Input: part model. Units: mm. Frame: model coordinates. A direction names the side the tool comes from. Give positions to 0.01 mm unless a question says otherwise; leave off trailing zeros. Loops run counter-clockwise (first coordinate to the right, second up) from the corner with the lowest first, then second, coordinate; pieces in that order, holes last. Notation, with made-up numbers: (47, -35) -> (77, -35) arc R15 ccw to (77, -17) -> close; hole circle Ø7 at (-7.75, 46.5). An arc over 180 degrees is marked (long way). Answer as a JSON object with one key per item and string values.
```python
from build123d import *

# Parameters (mm, degrees)
F0_R          = 10
F1_DEPTH      = 860
F2_R          = 20
F3_DEPTH      = 49.5
F4_R          = 3.75
F5_DEPTH      = 96
F5_DEPTH_BACK = 63
F6_R          = 17.5
F7_DEPTH      = 216
F8_R          = 7.8994
F9_DEPTH      = 850
F10_R         = 20
F10_R_2       = 10
F11_DEPTH     = 49
F12_R         = 17.5
F13_DEPTH     = 133


with BuildPart() as f1:
    # F0 (on Front) → F1 (new body)
    with BuildSketch(Plane.XZ):
        Circle(F0_R)
    extrude(amount=F1_DEPTH)

    # F2 (on Right) → F3 (join, symmetric)
    with BuildSketch(Plane.YZ):
        Circle(F2_R)
    extrude(amount=F3_DEPTH, both=True)

    # F4 (on Right) → F5 (cut, two sides)
    with BuildSketch(Plane.YZ) as f5_sk:
        with Locations((-722.5, 0)):
            Circle(F4_R)
    extrude(amount=F5_DEPTH, mode=Mode.SUBTRACT)
    extrude(f5_sk.sketch, amount=-F5_DEPTH_BACK, mode=Mode.SUBTRACT)

    # F6 (on face) → F7 (cut, symmetric)
    with BuildSketch(Plane.YZ.offset(49.5)):
        Circle(F6_R)
    extrude(amount=F7_DEPTH, both=True, mode=Mode.SUBTRACT)

    # F8 (on face) → F9 (cut)
    with BuildSketch(Plane.XZ.offset(860)):
        Circle(F8_R)
    extrude(amount=-F9_DEPTH, mode=Mode.SUBTRACT)

    # F10 (on Front) → F11 (join)
    with BuildSketch(Plane.XZ):
        Circle(F10_R)
        Circle(F10_R_2, mode=Mode.SUBTRACT)
    extrude(amount=F11_DEPTH)

    # F12 (on face) → F13 (cut)
    with BuildSketch(Plane.YZ.offset(49.5)):
        Circle(F12_R)
    extrude(amount=-F13_DEPTH, mode=Mode.SUBTRACT)


solid = f1.part
```
Q1. Access query for faces 5 (the cylindrical face through (9.54, -448.82, 3)), 6 (the cylindrical face through (0.693, 19.076, 6.007)), 7 (the flat face through (7, -860, -4)). Directions: +Z, -Z, +X, -X, +Y, -Y. A direction counts if a zero-diameter tool reaches every point of the face in a straight line with its end or side. Return the directions, or none.
Evaluation:
{"face 5": "-Y", "face 6": "none", "face 7": "+Z, -Z, +X, -X, -Y"}
Q2. Section A-A, the plane x = 39. Return the cut outline in (y, z), then the cut area to 3 significant figures.
Evaluation:
{"outline": "circle Ø40 at (0, 0); hole circle Ø35 at (0, 0)", "area": "295 mm2"}
Q3. Draft query along Z for faces 1 (the cylindrical face through (0.693, 16.166, -6.703)), 2 (the cylindrical face through (9.229, -29.601, -17.743)), 3 (the cylindrical face through (-1.712, -443.719, -7.712)), 4 (the flat face through (-5, -49, 9)). Return one class per face: +Z half, -Z half, draft (parallel to the pull), parting line (faces both ways), or undercut.
Evaluation:
{"face 1": "undercut", "face 2": "parting line", "face 3": "undercut", "face 4": "draft"}
Q4. Ray query, line 1 along Y through (x, z) = (11.5, 0); line 2 along X through (y, z) = (-519, 0); line 3 along X through (y, z) = (-682, -1). Return the intervals inside material, ascending.
Evaluation:
{"line 1": "y = -49 to -17.5, 17.5 to 20", "line 2": "x = -10 to -7.9, 7.9 to 10", "line 3": "x = -9.95 to -7.84, 7.84 to 9.95"}
Q5. Pin query (flat end, axial travel): pin 1 (4 mm diameter, centred on x = 3.5, z = 13, fed in from -Y); pin 2 (4 mm diameter, centred on x = 25, z = 11, fed in from +Y); pin 3 (10 mm diameter, centred on x = -10, y = -520.5, fed in from -Z). Return the tip coordinate at first contact, or that it passes through.
Evaluation:
{"pin 1": "stops at y = -49", "pin 2": "stops at y = 17.86", "pin 3": "stops at z = -8.66"}
Q6. Section B-B, the plane y = -487.5. Return the cut outline in (x, z).
Evaluation:
{"outline": "circle Ø20 at (0, 0); hole circle Ø15.8 at (0, 0)"}
